Can you work these out from the model? Positions are in its coordinate system, mm. A direction names the side the tool comes from. Round coordinates to 2 decimals unless told otherwise and drop trailing zeros. Loops run counter-clockwise (first coordinate to the right, second up) from the corner with the lowest first, then second, coordinate; pieces in that order, holes last. Notation, with made-up numbers: M 75,10.25 L 103,10.25 A12 ccw 103,33.25 Z; hole C 77.5,52 d11. An arc over 180 degrees is marked long. Answer as CSV lines item,"result".
from build123d import *

# Parameters (mm, degrees)
EXTRUDE_1_DEPTH     = 30
EXTRUDE_2_DEPTH     = 2
SKETCH_4_R          = 3
EXTRUDE_3_DEPTH     = 18
CUT_EXTRUDE_1_DEPTH = 6
SKETCH_6_W          = 12
SKETCH_6_H          = 4
EXTRUDE_4_DEPTH     = 2
CUT_EXTRUDE_2_DEPTH = 22
FILLET_1_R          = 2


with BuildPart() as part:
    # 스케치2 → 보스-돌출1 (new, symmetric)
    with BuildSketch(Plane(origin=(0, 0, 0), x_dir=(0, 0, -1), z_dir=(1, 0, 0))):
        Polygon((15.05, 0), (-15.05, 0), (-15.05, -30), (-19.05, -30), (-19.05, 0), (-30, 0), (-30, 8), (30, 8), (30, 0), (19.05, 0), (19.05, -30), (15.05, -30), align=None)
    extrude(amount=EXTRUDE_1_DEPTH, both=True)

    # 스케치3 → 보스-돌출2 (add, symmetric)
    with BuildSketch(Plane(origin=(0, 0, 0), x_dir=(0, 0, -1), z_dir=(1, 0, 0))):
        Polygon((-19.05, 0), (-27.05, 0), (-19.05, -24), align=None)
        Polygon((19.05, 0), (27.05, 0), (19.05, -24), align=None)
    extrude(amount=EXTRUDE_2_DEPTH, both=True)

    # 스케치4 → 보스-돌출3 (add, symmetric)
    with BuildSketch(Plane(origin=(0, 0, 0), x_dir=(0, 0, -1), z_dir=(1, 0, 0))):
        with BuildLine():
            Line((-6.421611649, 23.874648865), (-16, 8))
            Line((-16, 8), (16, 8))
            Line((16, 8), (6.421611649, 23.874648865))
            ThreePointArc((6.421611649, 23.874648865), (0, 27.5), (-6.421611649, 23.874648865))
        make_face()
        with Locations((0, 20)):
            Circle(SKETCH_4_R, mode=Mode.SUBTRACT)
    extrude(amount=EXTRUDE_3_DEPTH, both=True)

    # 스케치5 → 컷-돌출1 (cut, symmetric)
    with BuildSketch(Plane(origin=(0, 0, 0), x_dir=(0, 0, -1), z_dir=(1, 0, 0))):
        with BuildLine():
            Line((-6.421611649, 23.874648865), (-16, 8))
            Line((-16, 8), (16, 8))
            Line((16, 8), (6.421611649, 23.874648865))
            ThreePointArc((6.421611649, 23.874648865), (0, 27.5), (-6.421611649, 23.874648865))
        make_face()
    extrude(amount=CUT_EXTRUDE_1_DEPTH, both=True, mode=Mode.SUBTRACT)

    # 스케치6 → 보스-돌출4 (add, symmetric)
    with BuildSketch(Plane.XY):
        Polygon((-18, 8), (-22, 8), (-18, 12), align=None)
        with Locations((0, 10)):
            Rectangle(SKETCH_6_W, SKETCH_6_H)
        Polygon((17.991556012, 8), (18, 12), (21.991556012, 8), align=None)
    extrude(amount=EXTRUDE_4_DEPTH, both=True)

    # 스케치7 → 컷-돌출2 (cut, symmetric)
    with BuildSketch(Plane.XY):
        with BuildLine():
            Line((-19.5, -15), (-19.5, -30))
            Line((-19.5, -30), (-12.5, -30))
            Line((-12.5, -30), (-12.5, -15))
            ThreePointArc((-12.5, -15), (-16, -11.5), (-19.5, -15))
        make_face()
        with BuildLine():
            Line((12.5, -15), (12.5, -30))
            Line((12.5, -30), (19.5, -30))
            Line((19.5, -30), (19.5, -15))
            ThreePointArc((19.5, -15), (16, -11.5), (12.5, -15))
        make_face()
    extrude(amount=CUT_EXTRUDE_2_DEPTH, both=True, mode=Mode.SUBTRACT)

    # 필렛1
    fillet_1_edges = [part.edges().sort_by_distance(p)[0] for p in [
        (30, -15, -19.05),
        (-30, -15, 19.05),
        (-30, 4, 30),
        (-30, 8, 0),
        (0, -30, 19.05),
        (-24.75, -30, 19.05),
        (-30, 4, -30),
        (0, -30, -19.05),
        (-24.75, -30, -19.05),
        (-30, -15, -19.05),
        (30, 4, -30),
        (30, 8, 0),
        (24.75, -30, 19.05),
        (0, 0, 30),
        (0, 8, 30),
        (0, 8, -30),
        (0, 0, -30),
        (24.75, -30, -19.05),
        (30, 4, 30),
        (30, -15, 19.05),
    ]]
    fillet(fillet_1_edges, radius=FILLET_1_R)


solid = part.part
Item 1: If we section it at B-B on x = -16: Write out the boundary of the cut face in (y, z).
Output:
outline,"M -11.5,-19.05 L 0,-19.05 L 0,-28 A2 ccw 2,-30 L 6,-30 A2 ccw 8,-28 L 8,-16 L 23.87,-6.42 A7.5 ccw 23.87,6.42 L 8,16 L 8,28 A2 ccw 6,30 L 2,30 A2 ccw 0,28 L 0,19.05 L -11.5,19.05 L -11.5,15.05 L 0,15.05 L 0,-15.05 L -11.5,-15.05 Z; hole C 20,0 d6"
Item 2: We'd pull the mould along X, two halves only. Please class faces 1 (the face through (29.43, -15.21, -18.45)), 2 (the face through (19, 9, -2)), 3 (the face through (-19.5, -22, -17)): released by +X, released by -X, zero draft, split by the parting line, or undercut.
Output:
face 1,"released by +X"
face 2,"zero draft"
face 3,"undercut"
Item 3: If we section it at D-D on z = 21: Write out the boundary of the cut face in (x, y).
Output:
outline,"M -30,0 L -2,0 L -2,-18.15 L 2,-18.15 L 2,0 L 30,0 L 30,6 A2 ccw 28,8 L -28,8 A2 ccw -30,6 Z"
Item 4: Will these pins go through, and if not, where does the flat tip stop? pin 1 (9 mm diameter, centred on x = 0.5, y = -18, fed in from -Z); pin 2 (6 mm diameter, centred on y = 16, z = -6, fed in from -X); pin 3 (24 mm diameter, centred on x = -14.5, z = -1.5, fed in from -Y).
Output:
pin 1,"stops at z = -22.55"
pin 2,"stops at x = -18"
pin 3,"stops at y = 0"
Item 5: If we section it at C-C on y = -3.5: Write out the boundary of the cut face in (x, z), then the cut area to 3 significant figures.
Output:
outline,"M -30,-17.05 A2 ccw -28,-19.05 L -2,-19.05 L -2,-25.88 L 2,-25.88 L 2,-19.05 L 28,-19.05 A2 ccw 30,-17.05 L 30,-15.05 L -30,-15.05 Z; M -30,15.05 L 30,15.05 L 30,17.05 A2 ccw 28,19.05 L 2,19.05 L 2,25.88 L -2,25.88 L -2,19.05 L -28,19.05 A2 ccw -30,17.05 Z"
area,"531 mm2"
Item 6: If I drill on line 1 along Y through (x, z) = (12.75, 0); line 2 along Z through (x, y) = (9, -2); line 3 along X through (y, z) = (-3, -22), over which ranges is the centre line in solid material (lowest first)? Write a range as from..to.
Output:
line 1,"y = 0..17, 23..27.5"
line 2,"z = -19.05..-15.05, 15.05..19.05"
line 3,"x = -2..2"
Item 7: If we section it at A-A on z = 0: Write out the boundary of the cut face in (x, y), then the cut area to 3 significant figures.
Output:
outline,"M -30,0 L 30,0 L 30,6 A2 ccw 28,8 L 21.99,8 L 18,12 L 18,17 L 6,17 L 6,12 L -6,12 L -6,17 L -18,17 L -18,12 L -22,8 L -28,8 A2 ccw -30,6 Z; M -18,23 L -6,23 L -6,27.5 L -18,27.5 Z; M 6,23 L 18,23 L 18,27.5 L 6,27.5 Z"
area,"866 mm2"
Item 8: On a 3-axis mill with a long thin cutter (end or side, diameter ignored), from which of +Z, -Z, +X, -X, +Y, -Y can I reach the whole of each face in a straight line? I mean faces 4 (the face through (-2, -6, 21)), 5 (the face through (29.43, -14.79, 18.45)), 6 (the face through (-6, 16, 0)), 7 (the face through (0, -15, 15.05)). Say none if no direction works.
Output:
face 4,"+Z, -X, -Y"
face 5,"+Z, +X, -Y"
face 6,"+Y"
face 7,"+X, -X, -Y"
